Part print with two shaded views. Sizes in mm from the minimum x, y, z corner. A direction names the side the tool comes from. Round coordinates to 2 decimals unless told otherwise and drop trailing zeros. Loops run counter-clockwise (first coordinate to the right, second up) from the corner with the lowest first, then second, coordinate; pieces in that order, holes last. Notation, with made-up numbers: M 34,62.25 L 84,62.25 A17 cw 84,77.25 Z; hole C 80,38 d9. An arc over 180 degrees is marked long. Answer as CSV lines item,"result". Start each with the question number.
Item 1: Drop flat-ended pins along their axis: pin 1 Ø3 at (x, z) = (79, 5.5) entering from +Y; pin 2 Ø7.5 at (y, z) = (19, 9.5) entering from +X; pin 3 Ø2 at (y, z) = (16.5, 5) entering from -X. Give the stop position or say it passes through.
Item 2: Band-saw the part on C-C (y = 9). Give the cut face in (x, z), and give its area (3 significant figures).
Item 3: Band-saw the part on B-B (x = 40). Give the cut face in (y, z).
Item 4: Band-saw the part on A-A (z = 10). Give the cut face in (x, y).
Item 5: Which spindle directions (+Z, -Z, +X, -X, +Y, -Y) get a long thin tool onto all of the face, cutting with end or side? Do the marked faces 1, 2, 3, 4 and 5. Say none if no direction does.
Item 6: Wall check: line 1 (X direction, y = 29.5, z = 17.75); line 2 (Y direction, x = 42, z = 18.4); line 3 (Z direction, x = 10, y = 2). Give the ranges that are in metal, low to high.
Item 7: Mould opens along X. For the marked faces 6, 7 and 8 say: pulls with the +X half, pulls with the -X half, needs draft (parallel to the pull), parting line crosses it, or undercut.
Item 8: Band-saw the part on D-D (x = 60). Give the cut face in (y, z).
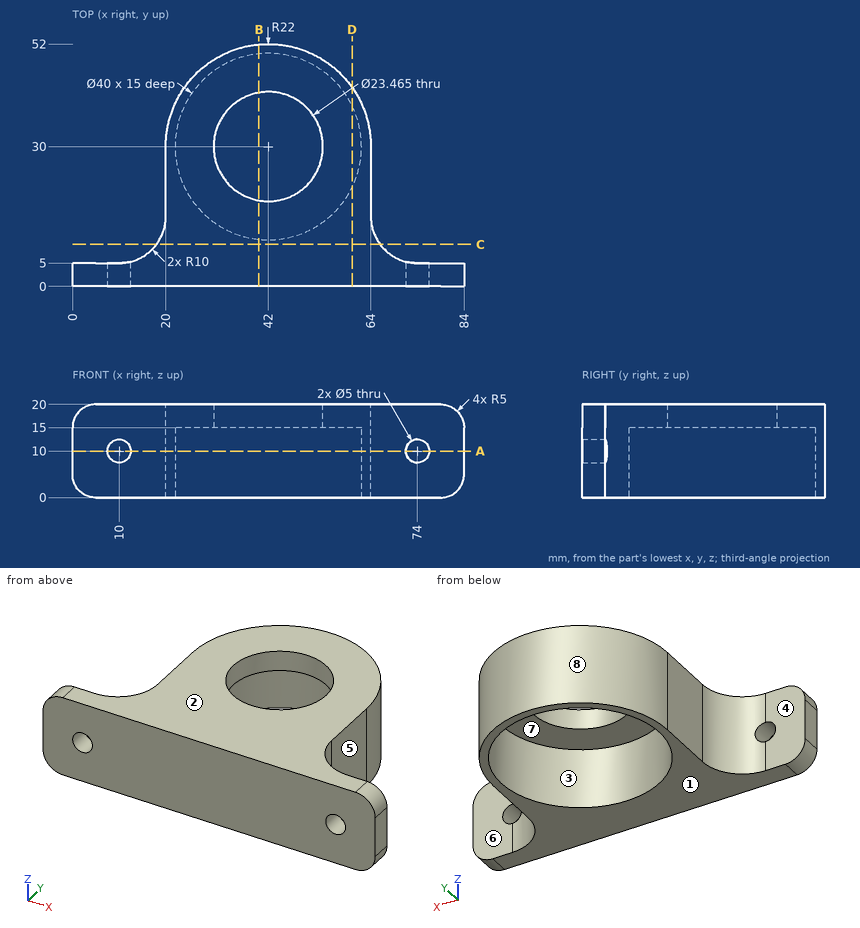
Answer block:
1,pin 1,"stops at y = 5"
1,pin 2,"stops at x = 64"
1,pin 3,"stops at x = 20"
2,outline,"M 18,0 L 66,0 L 66,20 L 18,20 Z"
2,area,"960 mm^2"
3,outline,"M 0,0 L 10.1,0 L 10.1,15 L 18.44,15 L 18.44,20 L 0,20 Z; M 41.56,15 L 49.9,15 L 49.9,0 L 51.91,0 L 51.91,20 L 41.56,20 Z"
4,outline,"M 0,0 L 7.5,0 L 7.5,5 L 0,5 Z; M 12.5,0 L 71.5,0 L 71.5,5.32 A10 cw 64,15 L 64,30 A22 ccw 20,30 L 20,15 A10 cw 12.5,5.32 Z; M 76.5,0 L 84,0 L 84,5 L 76.5,5 Z; hole C 42,30 d40"
5,face 1,"-Z, +X, -X, +Y, -Y"
5,face 2,"+Z, +X, -X, +Y, -Y"
5,face 3,"-Z"
5,face 4,"+Z, -Z, -X, +Y"
5,face 5,"+Z, -Z, +X, +Y"
6,line 1,"x = 20 to 30.28, 53.72 to 64"
6,line 2,"y = 0 to 18.27, 41.73 to 52"
6,line 3,"z = 0 to 7.5, 12.5 to 20"
7,face 6,"needs draft"
7,face 7,"undercut"
7,face 8,"parting line crosses it"
8,outline,"M 0,0 L 21.28,0 L 21.28,15 L 38.72,15 L 38.72,0 L 42.65,0 L 42.65,20 L 0,20 Z"
